from build123d import *

# Parameters (mm, degrees)
BOSS_EXTRUDE1_DEPTH = 170
SKETCH3_R           = 62.5
BOSS_EXTRUDE2_DEPTH = 75
SKETCH4_W           = 150
SKETCH4_H           = 150
BOSS_EXTRUDE3_DEPTH = 225
CUT_EXTRUDE6_DEPTH  = 225
SKETCH7_W           = 190
SKETCH7_H           = 20
BOSS_EXTRUDE5_DEPTH = 170
SKETCH10_W          = 150
SKETCH10_H          = 150
BOSS_EXTRUDE7_DEPTH = 225
CUT_EXTRUDE7_DEPTH  = 225
SKETCH12_R          = 75
SKETCH12_R_2        = 62.5
BOSS_EXTRUDE8_DEPTH = 75
BOSS_EXTRUDE9_START = -10
SKETCH13_R          = 67.5
SKETCH13_R_2        = 62.5
BOSS_EXTRUDE9_DEPTH = 10
SKETCH14_W          = 10
SKETCH14_H          = 14.038601632


with BuildPart() as part:
    # Sketch2 → Boss-Extrude1 (new body)
    with BuildSketch(Plane.XY):
        Polygon((-40.398264296, 30.238450413), (-20.398264296, 30.238450413), (-20.398264296, -139.761549587), (149.601735704, -139.761549587), (149.601735704, -159.761549587), (-40.398264296, -159.761549587), align=None)
    extrude(amount=-BOSS_EXTRUDE1_DEPTH)

    # Sketch3 → Boss-Extrude2 (add)
    with BuildSketch(Plane.ZY.offset(40.398264296)):
        with Locations((-85.93846623, -54.761549587)):
            Circle(SKETCH3_R)
    extrude(amount=BOSS_EXTRUDE2_DEPTH)

    # Sketch4 → Boss-Extrude3 (add)
    with BuildSketch(Plane(origin=(-20.398264296, 0, 0), x_dir=(0, 0, -1), z_dir=(1, 0, 0))):
        with Locations((85, -54.761549587)):
            Rectangle(SKETCH4_W, SKETCH4_H)
    extrude(amount=BOSS_EXTRUDE3_DEPTH)

    # Sketch5 → Cut-Extrude6 (cut)
    with BuildSketch(Plane(origin=(204.601735704, 0, 0), x_dir=(0, 0, -1), z_dir=(1, 0, 0))):
        with BuildLine():
            Line((35, 20.238450413), (10, 20.238450413))
            Line((10, 20.238450413), (10, -4.761549587))
            ThreePointArc((10, -4.761549587), (27.67766953, 2.560780883), (35, 20.238450413))
        make_face()
        with BuildLine():
            ThreePointArc((35, -129.761549587), (27.67766953, -112.083880057), (10, -104.761549587))
            Line((10, -104.761549587), (10, -129.761549587))
            Line((10, -129.761549587), (35, -129.761549587))
        make_face()
        with BuildLine():
            ThreePointArc((160, -104.761549587), (142.32233047, -112.083880057), (135, -129.761549587))
            Line((135, -129.761549587), (160, -129.761549587))
            Line((160, -129.761549587), (160, -104.761549587))
        make_face()
        with BuildLine():
            Line((160, 20.238450413), (135, 20.238450413))
            ThreePointArc((135, 20.238450413), (142.32233047, 2.560780883), (160, -4.761549587))
            Line((160, -4.761549587), (160, 20.238450413))
        make_face()
    extrude(amount=-CUT_EXTRUDE6_DEPTH, mode=Mode.SUBTRACT)

    # Sketch7 → Boss-Extrude5 (add)
    with BuildSketch(Plane.XZ.offset(159.761549587)):
        with Locations((54.601735704, -10)):
            Rectangle(SKETCH7_W, SKETCH7_H)
    extrude(amount=BOSS_EXTRUDE5_DEPTH)

    # Sketch10 → Boss-Extrude7 (add)
    with BuildSketch(Plane.XY):
        with Locations((64.601735704, -244.761549587)):
            Rectangle(SKETCH10_W, SKETCH10_H)
    extrude(amount=BOSS_EXTRUDE7_DEPTH)

    # Sketch11 → Cut-Extrude7 (cut)
    with BuildSketch(Plane.XY.offset(225)):
        with BuildLine():
            Line((14.601735704, -169.761549587), (-10.398264296, -169.761549587))
            Line((-10.398264296, -169.761549587), (-10.398264296, -194.761549587))
            ThreePointArc((-10.398264296, -194.761549587), (7.279405234, -187.439219117), (14.601735704, -169.761549587))
        make_face()
        with BuildLine():
            Line((139.601735704, -169.761549587), (114.601735704, -169.761549587))
            ThreePointArc((114.601735704, -169.761549587), (121.924066175, -187.439219117), (139.601735704, -194.761549587))
            Line((139.601735704, -194.761549587), (139.601735704, -169.761549587))
        make_face()
        with BuildLine():
            ThreePointArc((139.601735704, -294.761549587), (121.924066175, -302.083880057), (114.601735704, -319.761549587))
            Line((114.601735704, -319.761549587), (139.601735704, -319.761549587))
            Line((139.601735704, -319.761549587), (139.601735704, -294.761549587))
        make_face()
        with BuildLine():
            ThreePointArc((14.601735704, -319.761549587), (7.279405234, -302.083880057), (-10.398264296, -294.761549587))
            Line((-10.398264296, -294.761549587), (-10.398264296, -319.761549587))
            Line((-10.398264296, -319.761549587), (14.601735704, -319.761549587))
        make_face()
    extrude(amount=-CUT_EXTRUDE7_DEPTH, mode=Mode.SUBTRACT)

    # Sketch12 → Boss-Extrude8 (add)
    with BuildSketch(Plane(origin=(0, 0, -20), x_dir=(-1, 0, 0), z_dir=(0, 0, -1))):
        with Locations(Location((-64.601735704, -244.761549587, 0), (0, 0, 180))):
            Circle(SKETCH12_R)
        with Locations((-64.601735704, -244.761549587)):
            Circle(SKETCH12_R_2, mode=Mode.SUBTRACT)
    extrude(amount=BOSS_EXTRUDE8_DEPTH)

    # Sketch13 → Boss-Extrude9 (add)
    with BuildSketch(Plane.ZY.offset(115.398264296).offset(BOSS_EXTRUDE9_START)):
        with Locations((-85.93846623, -54.761549587)):
            Circle(SKETCH13_R)
        with Locations((-85.93846623, -54.761549587)):
            Circle(SKETCH13_R_2, mode=Mode.SUBTRACT)
    extrude(amount=BOSS_EXTRUDE9_DEPTH)

    # Sketch14 → Cut-Revolve1 (revolve, cut)
    with BuildSketch(Plane(origin=(64.601735704, 0, 0), x_dir=(0, 0, -1), z_dir=(1, 0, 0)), mode=Mode.PRIVATE) as cut_revolve1_sk:
        with Locations((25, -184.280850403)):
            Rectangle(SKETCH14_W, SKETCH14_H)
    revolve(cut_revolve1_sk.sketch.rotate(Axis((64.601735704, -244.761549587, -95), (0, 0, 1)), 90), axis=Axis((64.601735704, -244.761549587, -95), (0, 0, 1)), mode=Mode.SUBTRACT)


solid = part.part
Input: part model. Units: mm. Frame: model coordinates. A direction names the side the tool comes from. Coordinates: 2 decimals unless noted, no trailing zeros. Loops run counter-clockwise (first coordinate to the right, second up) from the corner with the lowest first, then second, coordinate; pieces in that order, holes last. Notation, with made-up numbers: (86, 15.25) - (135, 15.25) arc R13 cw to (135, 37.25) - close; hole circle Ø4 at (43.25, 48). An arc over 180 degrees is marked (long way). Answer in a Markdown table with one row per item. Add a question column.
Item 1: Section query D-D on y = -39. Return the cut outline in (x, z), then the cut area to 3 significant figures.
Item 2: Section query C-C on x = 163. Return the cut outline in (y, z), then the cut area to 3 significant figures.
Item 3: Mould query, pull axis Y, two halves, no side actions, for faces 6 (the flat face through (64, -246, -20)), 7 (the flat face through (139.602, -245, 111)), 8 (the cylindrical face through (-110.328, -80.614, -23.586)). Classes: released by +Y, released by -Y, zero draft, split by the parting line, or undercut.
Item 4: Contact query for flat-ended pins moving along their axis: P1, Ø3, axis at x = 79, z = -73, coming from the -Y side; P2, Ø8, axis at x = 25, z = 141.5, coming from the +Y side; P3, Ø6, axis at x = 119.5, y = -97.5, coming from the -Z side. Output: stop coordinate, or through.
Item 5: Section query B-B on z = 187. Return the cut outline in (x, y).
Item 6: Line query: line 1 along X through (y, z) = (-254.5, 81); line 2 along Y through (x, z) = (106.5, 14); line 3 along Y through (x, z) = (140, -114). Output: solid intervals per line, ascending. Write a range as [from, to].
Item 7: Section query A-A on z = -81. Return the cut outline in (x, y).
Item 8: Access query for faces 1 (the flat face through (5, -176, 0)), 2 (the flat face through (56, -159.762, -94)), 3 (the cylindrical face through (9.324, -295.45, -56.975)), 4 (the cylindrical face through (122.12, -301.89, 114.08)), 5 (the flat face through (91, -55, -160)). Directions: +Z, -Z, +X, -X, +Y, -Y. A direction counts if a zero-diameter tool reaches every point of the face in a straight line with its end or side. Return the directions, or none.
Recorded:
| question | item | result |
|---|---|---|
| 1 | outline | (-115.4, -151.57) - (-105.4, -151.57) - (-105.4, -146.42) - (-40.4, -146.42) - (-40.4, -170) - (-20.4, -170) - (-20.4, -160) - (204.6, -160) - (204.6, -10) - (-20.4, -10) - (-20.4, 0) - (-40.4, 0) - (-40.4, -25.46) - (-105.4, -25.46) - (-105.4, -20.3) - (-115.4, -20.3) - close |
| 1 | area | 46,300 mm^2 |
| 2 | outline | (-129.76, -135) arc R25 cw to (-104.76, -160) - (-4.76, -160) arc R25 cw to (20.24, -135) - (20.24, -35) arc R25 cw to (-4.76, -10) - (-104.76, -10) arc R25 cw to (-129.76, -35) - close |
| 2 | area | 20,500 mm^2 |
| 3 | face 6 | undercut |
| 3 | face 7 | zero draft |
| 3 | face 8 | split by the parting line |
| 4 | P1 | y = -318.64 |
| 4 | P2 | y = -169.76 |
| 4 | P3 | z = -160 |
| 5 | outline | (-10.4, -294.76) arc R25 cw to (14.6, -319.76) - (114.6, -319.76) arc R25 cw to (139.6, -294.76) - (139.6, -194.76) arc R25 cw to (114.6, -169.76) - (14.6, -169.76) arc R25 cw to (-10.4, -194.76) - close |
| 6 | line 1 | [-10.4, 139.6] |
| 6 | line 2 | [-319.76, -169.76] |
| 6 | line 3 | [-159.76, -139.76], [-129.76, 20.24] |
| 7 | outline | (-115.4, -122.08) - (-105.4, -122.08) - (-105.4, -117.07) - (-40.4, -117.07) - (-40.4, -159.76) - (149.6, -159.76) - (149.6, -139.76) - (-20.4, -139.76) - (-20.4, -129.76) - (204.6, -129.76) - (204.6, 20.24) - (-20.4, 20.24) - (-20.4, 30.24) - (-40.4, 30.24) - (-40.4, 7.54) - (-105.4, 7.54) - (-105.4, 12.56) - (-115.4, 12.56) - close; circle Ø150 at (64.6, -244.76); hole circle Ø125 at (64.6, -244.76) |
| 8 | face 1 | +Z |
| 8 | face 2 | -Z, +X, -X |
| 8 | face 3 | -Z |
| 8 | face 4 | +Z, +X, -Y |
| 8 | face 5 | -Z, +X, +Y |
